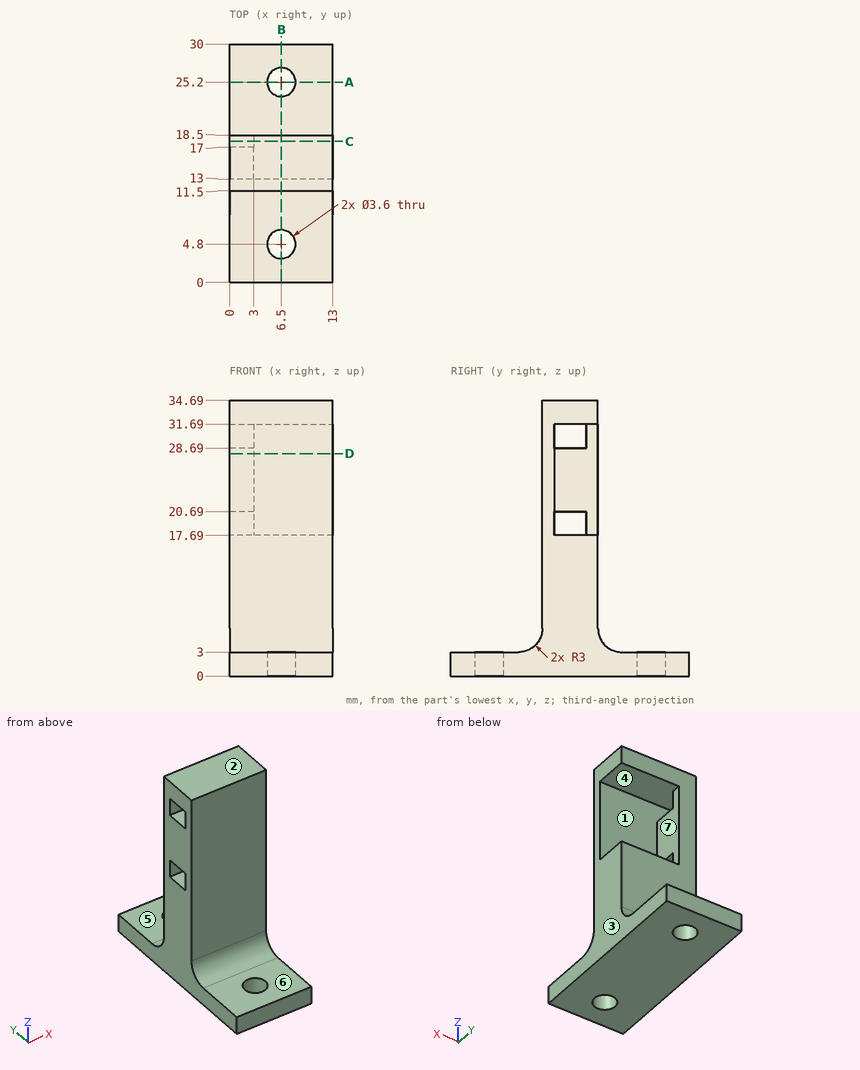
The drawing under review shows one solid part. Ordinate dimensions are in mm from its lowest x, y, z. A direction names the side the tool comes from. Round coordinates to 2 decimals unless told otherwise and drop trailing zeros. Order: outer loops, then holes, each group sorted by start corner. A loop starts at its lowest first (then second) coordinate and runs counter-clockwise, first axis right, second up. Notation, with made-up numbers: (-34.75, 10.25) - (10.25, 10.25) arc R32 cw to (10.25, 41.25) - close; hole circle Ø5 at (3.5, 65.5). An arc over 180 degrees is marked (long way). Return JSON: item names as keys, results as strings.
Q1. Consider section D-D on z = 28. Write out the cut boundary in (x, y), plus the area to 3 significant figures.
Computed values:
{"outline": "(0, 11.5) - (13, 11.5) - (13, 13) - (3, 13) - (3, 18.5) - (0, 18.5) - close", "area": "36.0 mm2"}
Q2. For pin 1 Ø6.5 at (x, z) = (4, 26.5) entering from -Y; pin 2 Ø4 at (x, z) = (3, 22.5) entering from +Y; pin 3 Ø2.5 at (x, y) = (9, 26.5) entering from +Z, all flat-tipped, find the tip position at first contact; note any pin that passes through.
Computed values:
{"pin 1": "stops at y = 11.5", "pin 2": "stops at y = 18.5", "pin 3": "stops at z = 3"}
Q3. Wall thickness on L1, parallel to Y at x = 6.5, z = 1.8; L2, parallel to Z at x = 12.5, y = 17; L3, parallel to Y at x = 8, z = 2: over which ranges is each line inside the solid? List them lowest first. Write a range as [from, to].
Computed values:
{"L1": "y = [0, 3], [6.6, 23.4], [27, 30]", "L2": "z = [0, 17.69], [31.69, 34.69]", "L3": "y = [0, 3.81], [5.79, 24.21], [26.19, 30]"}
Q4. Consider section C-C on y = 17.75. Write out the cut boundary in (x, z), plus the area to 3 significant figures.
Computed values:
{"outline": "(0, 0) - (13, 0) - (13, 17.69) - (3, 17.69) - (3, 31.69) - (13, 31.69) - (13, 34.69) - (0, 34.69) - close", "area": "311 mm2"}
Q5. Consider section A-A on y = 25.2. Write out the cut boundary in (x, z), plus the area to 3 significant figures.
Computed values:
{"outline": "(0, 0) - (4.7, 0) - (4.7, 3) - (0, 3) - close; (8.3, 0) - (13, 0) - (13, 3) - (8.3, 3) - close", "area": "28.2 mm2"}
Q6. Machinability: for the marked faces 4, 5, 6 and 7, which of the approach directions +Z, -Z, +X, -X, +Y, -Y give a long, thin tool a straight path to every point of the face, cutting with its end or side? Answer none if there is none.
Computed values:
{"face 4": "+X", "face 5": "+Z, +X, -X, +Y", "face 6": "+Z, +X, -X, -Y", "face 7": "+X, +Y"}
Q7. Consider section B-B on x = 6.5. Write out the cut boundary in (y, z), plus the area to 3 significant figures.
Computed values:
{"outline": "(0, 0) - (3, 0) - (3, 3) - (0, 3) - close; (6.6, 0) - (23.4, 0) - (23.4, 3) - (21.5, 3) arc R3 cw to (18.5, 6) - (18.5, 17.69) - (13, 17.69) - (13, 31.69) - (18.5, 31.69) - (18.5, 34.69) - (11.5, 34.69) - (11.5, 6) arc R3 cw to (8.5, 3) - (6.6, 3) - close; (27, 0) - (30, 0) - (30, 3) - (27, 3) - close", "area": "217 mm2"}
Q8. The part is to be moulded in two halves that separate along Z. For the marked faces 1, 2 and 3, say which applies: pulls with the +Z half, pulls with the -Z half, needs draft (parallel to the pull), parting line crosses it, or undercut.
Computed values:
{"face 1": "undercut", "face 2": "pulls with the +Z half", "face 3": "needs draft"}
